The model under review builds one solid part; all positions refer to its coordinate system, in mm. Face numbers are marked on the shaded views. A direction names the side the tool comes from. Coordinates: 2 decimals unless noted, no trailing zeros. Order: outer loops, then holes, each group sorted by start corner. A loop starts at its lowest first (then second) coordinate and runs counter-clockwise, first axis right, second up. Notation, with made-up numbers: (36.25, 68.25) -> (87.25, 68.25) arc R21 ccw to (87.25, 94.25) -> close; hole circle Ø3 at (16.25, -9.75). An arc over 180 degrees is marked (long way). Use one line per item in the form item = value.
from build123d import *


with BuildPart() as part:
    # Croquis1 → Revolución1 (revolve)
    with BuildSketch(Plane.XY, mode=Mode.PRIVATE) as revoluci_n1_sk:
        Polygon((7.346100741, 8.5), (7.346100741, 35.5), (10.846100741, 35.5), (10.846100741, 33), (16.846100741, 33), (16.846100741, 39.5), (19.346100741, 39.5), (19.346100741, 37), (29.346100741, 37), (29.346100741, 39.5), (31.846100741, 39.5), (31.846100741, 33), (37.846100741, 33), (37.846100741, 35.5), (41.346100741, 35.5), (41.346100741, 8.5), align=None)
    revolve(revoluci_n1_sk.sketch.rotate(Axis((-1, 0.5, 0), (1, 0, 0)), 90), axis=Axis((-1, 0.5, 0), (1, 0, 0)))


solid = part.part
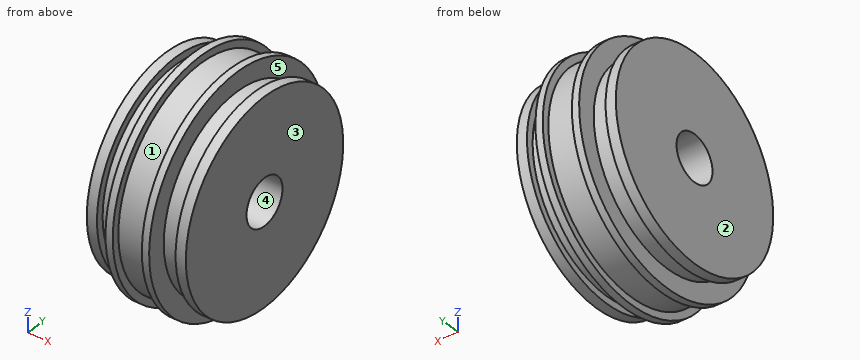
Item 1: Tool access review of the marked faces 1 and 2: name each direction out of +Z, -Z, +X, -X, +Y, -Y from which nothing blocks a thin tool from reaching the whole face with its end or side.
Results found:
face_1 = none
face_2 = +Z, -Z, -X, +Y, -Y
Item 2: To check wall thickness, follow L1, parallel to Y at x = 19, z = 0; L2, parallel to Z at x = 28, y = 0; L3, parallel to Y at x = 34, z = 0. State the ranges of each line that lie inside material, in increasing order. Write a range as from..to.
Results found:
L1 = -38.5..-7.5, 8.5..39.5
L2 = -36.5..-7.98, 7.98..36.5
L3 = -32..-7.5, 8.5..33
Item 3: Clearance check with flat-ended pins moving along their axes: pin 1 (9.5 mm diameter, centred on y = 0.5, z = 0, fed in from +X); pin 2 (1.5 mm diameter, centred on x = 37.5, z = -1, fed in from +Y); pin 3 (6 mm diameter, centred on x = 27.5, y = 25, fed in from +Z); pin 4 (3 mm diameter, centred on x = 35, z = -25, fed in from +Y). State where each tip first meets the part, or that it passes through.
Results found:
pin_1 = through
pin_2 = 35.5
pin_3 = 32.11
pin_4 = 22.95
Item 4: We need section C-C (z = 34). Write out the cut boundary in (x, y), plus the area to 3 significant figures.
Results found:
outline = (7.35, -7.81) -> (10.85, -7.81) -> (10.85, 8.81) -> (7.35, 8.81) -> close; (16.85, -18.6) -> (19.35, -18.6) -> (19.35, -12.78) -> (29.35, -12.78) -> (29.35, -18.6) -> (31.85, -18.6) -> (31.85, 19.6) -> (29.35, 19.6) -> (29.35, 13.78) -> (19.35, 13.78) -> (19.35, 19.6) -> (16.85, 19.6) -> close; (37.85, -7.81) -> (41.35, -7.81) -> (41.35, 8.81) -> (37.85, 8.81) -> close
area = 573 mm²
Item 5: We need section D-D (x = 22). Write out the cut boundary in (y, z), plus the area to 3 significant figures.
Results found:
outline = circle Ø73 at (0.5, 0); hole circle Ø16 at (0.5, 0)
area = 3,980 mm²
Item 6: Draft analysis for pull direction X (two halves, no side actions). For the marked faces 3, 4 and 5, state which applies: released by +X, released by -X, zero draft, split by the parting line, or undercut.
Results found:
face_3 = released by +X
face_4 = zero draft
face_5 = undercut
